Part model, mm, in its own coordinate system. Face numbers are marked on the shaded views. A direction names the side the tool comes from. Round coordinates to 2 decimals unless told otherwise and drop trailing zeros. Loops run counter-clockwise (first coordinate to the right, second up) from the corner with the lowest first, then second, coordinate; pieces in that order, holes last. Notation, with made-up numbers: M 30.25,47.25 L 85.25,47.25 A18 ccw 85.25,80.25 Z; hole C -33,61 d11. An arc over 180 degrees is marked long. Put each result on its own line as item: value. Start each with the question number.
1) Slice it at C-C on z = -12.5. Give the cut face in (x, y).
2) Slice it at A-A on x = 43.66. Give the cut face in (y, z).
3) Drop flat-ended pins along their axis: pin 1 Ø5 at (x, z) = (-54.66, -12.5) entering from +Y; pin 2 Ø4 at (x, y) = (-42.5, 7) entering from +Z. Give the stop position or say it passes through.
4) Probe line 1 along X through (y, z) = (7.25, -12.5); line 2 along Z through (x, y) = (43.66, 9); line 3 along Z through (x, y) = (73.5, 5). List the from-to ranges inside material, lowest first.
5) Slice it at D-D on x = -50.5. Give the cut face in (y, z).
6) Slice it at B-B on y = 2. State how many separate pieces and enclosed holes the cut face has, then the cut area to 3 significant figures.
7) Which spindle directions (+Z, -Z, +X, -X, +Y, -Y) get a long thin tool onto all of the face, cutting with end or side? Do the marked faces 1, 2 and 3. Say none if no direction does.
8) Pull direction Z, two halves, no side cores. Call the marked faces 4, 5 and 6: +Z half, -Z half, draft (parallel to the pull), parting line (faces both ways), or undercut.
```python
from build123d import *

# Parameters (mm, degrees)
SKETCH1_R            = 2.75
SKETCH1_W            = 20
SKETCH1_H            = 20
BOSS_EXTRUDE1_DEPTH  = 14.1
MOVE_FACE1_BY        = 20
SKETCH6_W            = 30.987343285
SKETCH6_H            = 33.189068773
BOSS_EXTRUDE2_DEPTH  = 14.1
M5_CLEARANCE_HOLE2_D = 5.5


with BuildPart() as part:
    # Sketch1 → Boss-Extrude1 (new body)
    with BuildSketch(Plane(origin=(0, 0, 0), x_dir=(1, 0, 0), z_dir=(0, 1, 0))):
        with BuildLine():
            Line((10, -22.5), (16.339745962, -22.5))
            ThreePointArc((16.339745962, -22.5), (20, -18.839745962), (25, -17.5))
            Line((25, -17.5), (64.66, -17.5))
            Line((64.66, -17.5), (64.66, 22.5))
            Line((64.66, 22.5), (-64.66, 22.5))
            Line((-64.66, 22.5), (-64.66, -17.5))
            Line((-64.66, -17.5), (-25, -17.5))
            ThreePointArc((-25, -17.5), (-20, -18.839745962), (-16.339745962, -22.5))
            Line((-16.339745962, -22.5), (-10, -22.5))
            Line((-10, -22.5), (10, -22.5))
        make_face()
        with Locations(Location((34.66, 12.5, 0), (0, 0, 270))):
            Circle(SKETCH1_R, mode=Mode.SUBTRACT)
        with Locations(Location((34.66, -7.5, 0), (0, 0, 270))):
            Circle(SKETCH1_R, mode=Mode.SUBTRACT)
        with Locations(Location((54.66, -7.5, 0), (0, 0, 270))):
            Circle(SKETCH1_R, mode=Mode.SUBTRACT)
        with Locations(Location((54.66, 12.5, 0), (0, 0, 270))):
            Circle(SKETCH1_R, mode=Mode.SUBTRACT)
        with Locations(Location((-54.66, -7.5, 0), (0, 0, 270))):
            Circle(SKETCH1_R, mode=Mode.SUBTRACT)
        with Locations(Location((-34.66, 12.5, 0), (0, 0, 270))):
            Circle(SKETCH1_R, mode=Mode.SUBTRACT)
        with Locations(Location((-54.66, 12.5, 0), (0, 0, 270))):
            Circle(SKETCH1_R, mode=Mode.SUBTRACT)
        with Locations(Location((-34.66, -7.5, 0), (0, 0, 270))):
            Circle(SKETCH1_R, mode=Mode.SUBTRACT)
        with Locations((0, -7.5)):
            Rectangle(SKETCH1_W, SKETCH1_H, mode=Mode.SUBTRACT)
    extrude(amount=BOSS_EXTRUDE1_DEPTH)

    # Move Face1: a face moved outward by 20.0
    extrude(part.faces().sort_by_distance((64.66, 7.05, -2.5))[0], amount=MOVE_FACE1_BY, dir=(1, 0, 0))

    # Sketch6 → Boss-Extrude2 (add)
    with BuildSketch(Plane.XZ):
        with Locations((43.846371015, -2.215029501)):
            Rectangle(SKETCH6_W, SKETCH6_H)
    extrude(amount=-BOSS_EXTRUDE2_DEPTH)

    # M5 Clearance Hole2 (through all)
    with Locations(Plane(origin=(0, 0, 0), x_dir=(-1, 0, 0), z_dir=(0, -1, 0))):
        with Locations((-74.66, -7.5), (-43.66, -7.5), (-43.66, 12.5), (-74.66, 12.5)):
            Hole(M5_CLEARANCE_HOLE2_D / 2)


solid = part.part
```
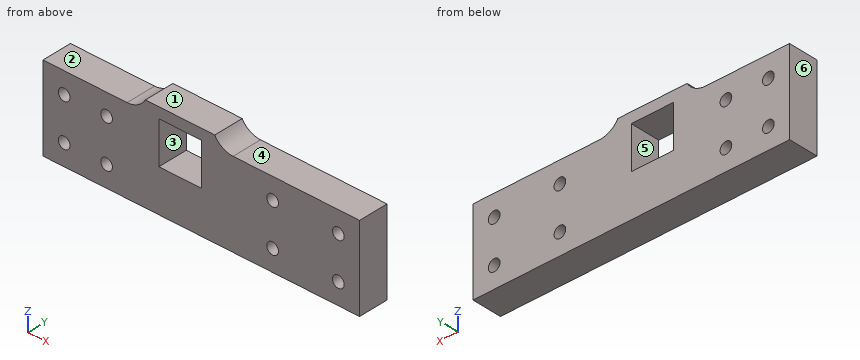
Recorded:
1. outline: M -64.66,0 L -57.41,0 L -57.41,14.1 L -64.66,14.1 Z; M -51.91,0 L -37.41,0 L -37.41,14.1 L -51.91,14.1 Z; M -31.91,0 L 40.91,0 L 40.91,14.1 L -31.91,14.1 Z; M 46.41,0 L 71.91,0 L 71.91,14.1 L 46.41,14.1 Z; M 77.41,0 L 84.66,0 L 84.66,14.1 L 77.41,14.1 Z
2. outline: M 0,-22.5 L 14.1,-22.5 L 14.1,-15.25 L 0,-15.25 Z; M 0,-9.75 L 14.1,-9.75 L 14.1,4.75 L 0,4.75 Z; M 0,10.25 L 14.1,10.25 L 14.1,17.5 L 0,17.5 Z
3. pin 1: passes through
3. pin 2: stops at z = 17.5
4. line 1: x = -64.66 to -57.41, -51.91 to -37.41, -31.91 to 40.91, 46.41 to 71.91, 77.41 to 84.66
4. line 2: z = -22.5 to -15.25, -9.75 to 4.75, 10.25 to 17.5
4. line 3: z = -22.5 to -14.99, -10.01 to 5.01, 9.99 to 17.5
5. outline: M 0,-22.5 L 14.1,-22.5 L 14.1,17.5 L 0,17.5 Z
6. separate pieces: 1
6. enclosed holes: 9
6. area: 5,570 mm2
7. face 1: +Z, +X, -X, +Y, -Y
7. face 2: +Z, -X, +Y, -Y
7. face 3: +Y, -Y
8. face 4: +Z half
8. face 5: undercut
8. face 6: draft
